The drawing under review shows one solid part. Ordinate dimensions are in mm from its lowest x, y, z. Coordinates: 2 decimals unless noted, no trailing zeros. Order: outer loops, then holes, each group sorted by start corner. A loop starts at its lowest first (then second) coordinate and runs counter-clockwise, first axis right, second up. Notation, with made-up numbers: (10, -33.5) -> (18, -33.5) arc R31 ccw to (18, -4.5) -> close; hole circle Ø11 at (86, 16.5). An arc over 180 degrees is marked (long way). Use one line per item in the form item = value.
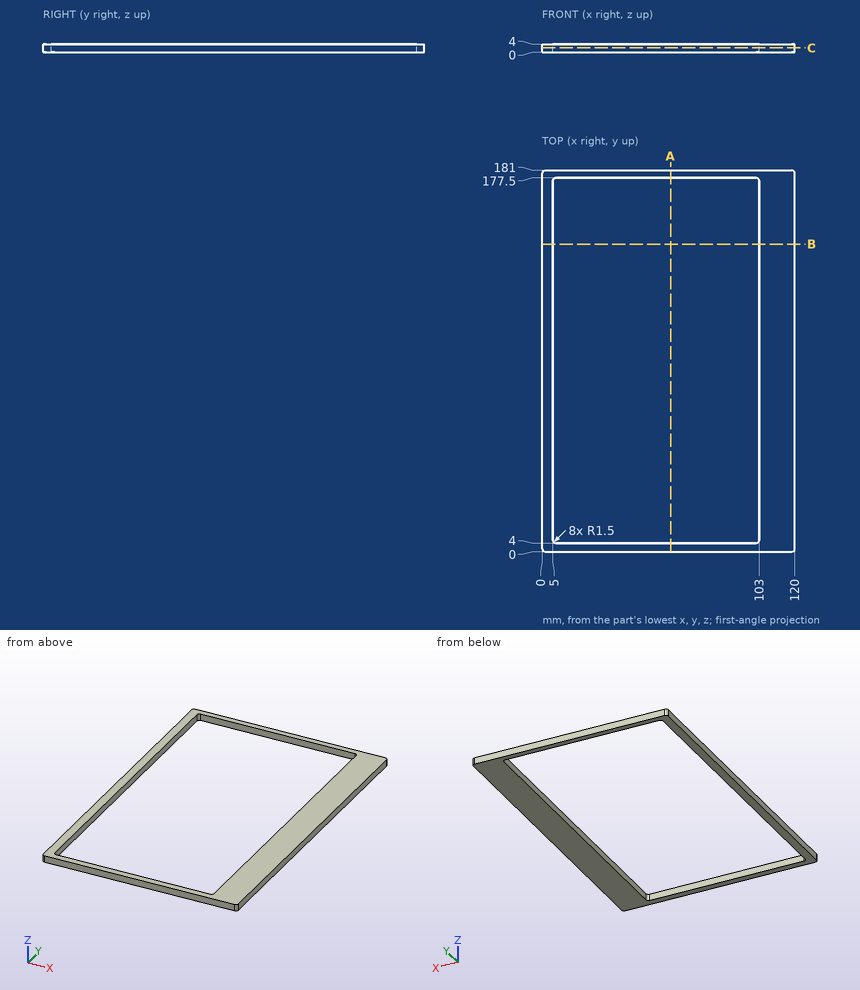
Item 1: We need section C-C (z = 2.2). Write out the cut boundary in (x, y).
Results found:
outline = (0, 1.5) arc R1.5 ccw to (1.5, 0) -> (118.5, 0) arc R1.5 ccw to (120, 1.5) -> (120, 179.5) arc R1.5 ccw to (118.5, 181) -> (1.5, 181) arc R1.5 ccw to (0, 179.5) -> close; hole (5, 5.5) arc R1.5 ccw to (6.5, 4) -> (101.5, 4) arc R1.5 ccw to (103, 5.5) -> (103, 176) arc R1.5 ccw to (101.5, 177.5) -> (6.5, 177.5) arc R1.5 ccw to (5, 176) -> close
Item 2: We need section A-A (x = 61). Write out the cut boundary in (y, z), plus the area to 3 significant figures.
Results found:
outline = (0, 0) -> (4, 0) -> (4, 4) -> (0, 4) -> close; (177.5, 0) -> (181, 0) -> (181, 4) -> (177.5, 4) -> close
area = 30.0 mm²
Item 3: We need section B-B (y = 146). Write out the cut boundary in (x, z).
Results found:
outline = (0, 0) -> (5, 0) -> (5, 4) -> (0, 4) -> close; (103, 0) -> (120, 0) -> (120, 4) -> (103, 4) -> close
Item 4: To check wall thickness, follow L1, parallel to Y at x = 47.5, z = 2.65; L2, parallel to X at y = 102, z = 2.75. State the ranges of each line that lie inside material, in increasing order. Write a range as from..to.
Results found:
L1 = 0..4, 177.5..181
L2 = 0..5, 103..120
